```python
from build123d import *

# Parameters (mm, degrees)
F1_ANGLE = 180


with BuildPart() as f1:
    # F0 (on Top) → F1 (revolve)
    with BuildSketch(Plane.XY):
        Polygon((107.95, 19.05), (101.6, 19.05), (101.6, 0), (114.3, 0), (114.3, 12.7), align=None)
    revolve(axis=Axis((0, 5.0604422272, 0), (0, -1, 0)), revolution_arc=F1_ANGLE)

    # F2: F1 across plane


with BuildPart() as f1_1:
    add(f1.part)
    add(f1.part.mirror(Plane.XZ))


solid = f1_1.part
```
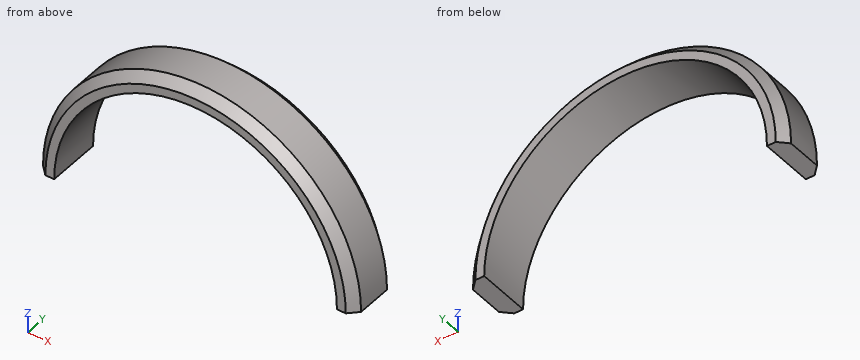
Verification items for the finished model (mm, model axes). Round coordinates to 2 decimals unless told otherwise and drop trailing zeros. Write each loop counter-clockwise with the first axis right and the second up, starting at its lowest first coordinate (ties: lowest second). Pieces come first, ordered by that corner, then holes. Notation, with made-up numbers: (74, 43.25) -> (121, 43.25) arc R22 ccw to (121, 78.25) -> close; hole circle Ø10 at (87, -19). An arc over 180 degrees is marked (long way). Write each question's results on one line, items separated by ' | '. Start each with the question number.
1. Material ranges on probe 1 along X at (y, z) = (16, 17.5); probe 2 along X at (y, z) = (-8.5, 39); probe 3 along Z at (x, y) = (86, -8), recorded low to high. Write a range as from..to.
2. Cross-section at A-A (x = 0). Enter the section's corners in (y, z).
3. Cross-section at B-B (y = -7.5). Enter the section's corners in (x, z).
4. Depth check by flat-ended pin: P1, Ø3, axis at x = -32.5, y = 0.5, coming from the +Z side; P2, Ø1.5, axis at x = 16, y = -8, coming from the +Z side; P3, Ø4, axis at x = 63.5, y = 5.5, coming from the +Z side. Enter the tip coordinate at first touch or a pass-through.
Solutions:
1) probe 1: x = -109.61..-100.08, 100.08..109.61 | probe 2: x = -107.44..-93.82, 93.82..107.44 | probe 3: z = 54.1..75.29
2) outline: (-19.05, 101.6) -> (19.05, 101.6) -> (19.05, 107.95) -> (12.7, 114.3) -> (-12.7, 114.3) -> (-19.05, 107.95) -> close
3) outline: (-114.3, 0) -> (-101.6, 0) arc R101.6 cw to (101.6, 0) -> (114.3, 0) arc R114.3 ccw to start
4) P1: stops at z = 110.02 | P2: stops at z = 113.28 | P3: stops at z = 96.34
